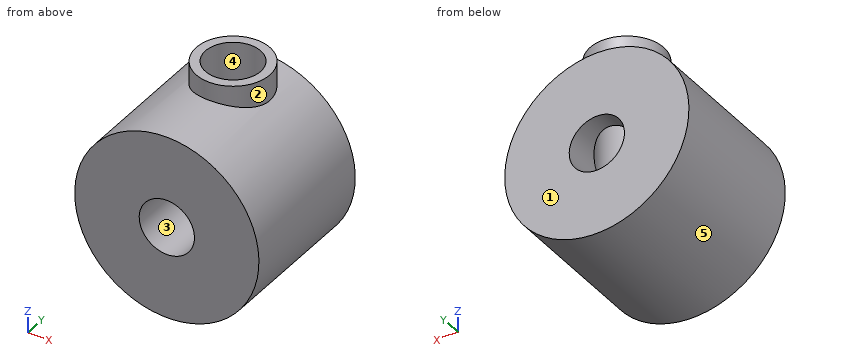
from build123d import *

# Parameters (mm, degrees)
SKETCH1_R               = 5
SKETCH1_R_2             = 1.5
BOSS_EXTRUDE1_DEPTH     = 8
SKETCH6_R               = 2
BOSS_EXTRUDE4_DEPTH     = 3.5
CUT_EXTRUDE3_REACH      = 16.491
CUT_EXTRUDE3_END_RADIUS = 1.5
SKETCH7_R               = 1.5


with BuildPart() as part:
    # Sketch1 → Boss-Extrude1 (new body)
    with BuildSketch(Plane(origin=(0, 0, 0), x_dir=(1, 0, 0), z_dir=(0, 1, 0))):
        with Locations(Location((0, 0, 0), (0, 0, 270))):
            Circle(SKETCH1_R)
        with Locations(Location((0, 0, 0), (0, 0, 270))):
            Circle(SKETCH1_R_2, mode=Mode.SUBTRACT)
    extrude(amount=BOSS_EXTRUDE1_DEPTH)

    # Sketch6 → Boss-Extrude4 (add)
    with BuildSketch(Plane.XY.offset(6)):
        with Locations((0, 5.5)):
            Circle(SKETCH6_R)
    extrude(amount=-BOSS_EXTRUDE4_DEPTH)

    # Cut-Extrude3: up to this cylinder (the profile starts outside it)
    cut_extrude3_end = Plane(origin=(0, 5.5, 0), z_dir=(0, -1, 0)) * Cylinder(CUT_EXTRUDE3_END_RADIUS, 36.982, mode=Mode.PRIVATE)
    # Sketch7 → Cut-Extrude3 (cut, up to the surface)
    with BuildSketch(Plane.XY.offset(6), mode=Mode.PRIVATE) as cut_extrude3_sk1:
        with Locations((0, 5.5)):
            Circle(SKETCH7_R)
    cut_extrude3_tool1 = extrude(cut_extrude3_sk1.sketch, amount=-CUT_EXTRUDE3_REACH, mode=Mode.PRIVATE) - cut_extrude3_end
    add(cut_extrude3_tool1.solids().sort_by_distance((0, 5.5, 6))[0], mode=Mode.SUBTRACT)


solid = part.part
Design review of the part built by this model. Coordinates are the model's own, in mm. Face numbers are marked on the shaded views. A direction names the side the tool comes from. Coordinates: 2 decimals unless noted, no trailing zeros. Order: outer loops, then holes, each group sorted by start corner. A loop starts at its lowest first (then second) coordinate and runs counter-clockwise, first axis right, second up. Notation, with made-up numbers: (30.25, 16.5) - (53.25, 16.5) arc R30 cw to (53.25, 42.5) - close; hole circle Ø10 at (44.5, 76). An arc over 180 degrees is marked (long way). Put each result on its own line as item: value.
1) Take a section at D-D, the plane z = 5.25. Give the boundary of the cut face in (x, y).
Response values:
outline: circle Ø4 at (0, 5.5); hole circle Ø3 at (0, 5.5)
2) Take a section at C-C, the plane z = -0.5. Give the boundary of the cut face in (x, y).
Response values:
outline: (-4.97, 0) - (-1.41, 0) - (-1.41, 8) - (-4.97, 8) - close; (1.41, 0) - (4.97, 0) - (4.97, 8) - (1.41, 8) - close
3) The part is to be moulded in two halves that separate along Z. For the marked faces 3, 4 and 5, say which applies: released by +Z, released by -Z, zero draft, split by the parting line, or undercut.
Response values:
face 3: undercut
face 4: zero draft
face 5: split by the parting line
4) Wall thickness on L1, parallel to X at y = 3, z = 0; L2, parallel to X at y = 5.5, z = 4.85; L3, parallel to Y at x = 0, z = 4.65: over which ranges is each line inside the solid? List them lowest first. Write a range as from..to.
Response values:
L1: x = -5..-1.5, 1.5..5
L2: x = -2..-1.5, 1.5..2
L3: y = 0..4, 7..8
5) Take a section at A-A, the plane x = 0. Give the boundary of the cut face in (y, z).
Response values:
outline: (0, -5) - (8, -5) - (8, -1.5) - (0, -1.5) - close; (0, 1.5) - (4, 1.5) - (4, 6) - (3.5, 6) - (3.5, 5) - (0, 5) - close; (7, 1.5) - (8, 1.5) - (8, 5) - (7.5, 5) - (7.5, 6) - (7, 6) - close
6) Tool access review of the marked faces 1 and 2: name each direction out of +Z, -Z, +X, -X, +Y, -Y from which nothing blocks a thin tool from reaching the whole face with its end or side.
Response values:
face 1: +Z, -Z, +X, -X, +Y
face 2: +Z
7) Insertion check: P1, Ø3, axis at y = 5.5, z = -1.5, coming from the -X side. The pin has a flat end and moves straight along its axis. Give the tip position at first contact, or say it passes through.
Response values:
P1: stops at x = -5
8) Take a section at B-B, the plane y = 5.5. Give the boundary of the cut face in (x, z), and give its area (3 significant figures).
Response values:
outline: (-2, 4.58) arc R5 ccw (long way) to (2, 4.58) - (2, 6) - (1.5, 6) - (1.5, 0) arc R1.5 cw to (-1.5, 0) - (-1.5, 6) - (-2, 6) - close
area: 61.6 mm²
